Could you check a few things on this model? Use its own coordinates, in mm. Face numbers are marked on the shaded views. A direction names the side the tool comes from. Round coordinates to 2 decimals unless told otherwise and drop trailing zeros. Write each loop counter-clockwise with the first axis right and the second up, starting at its lowest first coordinate (ties: lowest second). Pieces come first, ordered by that corner, then holes. Notation, with made-up numbers: (-31, -18.5) -> (-10, -18.5) arc R13 cw to (-10, -4.5) -> close; hole circle Ø9 at (-30, 34). An arc over 180 degrees is marked (long way). Answer in a Markdown table with one row per item.
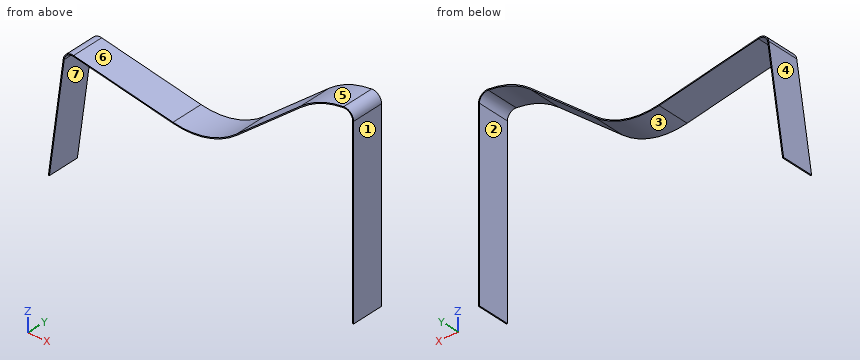
from build123d import *

# Parameters (mm, degrees)
F1_DEPTH      = 25.4
F1_DEPTH_BACK = 25.4


with BuildPart() as f1:
    # F0 (on Front) → F1 (new body, two sides)
    with BuildSketch(Plane.XZ) as f1_sk:
        with BuildLine():
            Line((-1.560986, 0.208131), (0, 0))
            Line((0, 0), (23.665896, 177.494217))
            ThreePointArc((23.665896, 177.494217), (28.705317, 186.028474), (38.342357, 188.34294))
            Line((38.342357, 188.34294), (196.490305, 161.984949))
            ThreePointArc((196.490305, 161.984949), (250.659549, 164.697858), (298.757135, 189.763554))
            Line((298.757135, 189.763554), (401.211842, 275.293424))
            ThreePointArc((401.211842, 275.293424), (432.73779, 294.602226), (468.488889, 304.013615))
            ThreePointArc((468.488889, 304.013615), (478.366667, 300.858274), (482.6, 291.392253))
            Line((482.6, 291.392253), (482.6, 0))
            Line((482.6, 0), (484.1748, 0))
            Line((484.1748, 0), (484.1748, 291.392253))
            ThreePointArc((484.1748, 291.392253), (479.416533, 302.032061), (468.313911, 305.578664))
            ThreePointArc((468.313911, 305.578664), (432.119499, 296.050574), (400.202629, 276.502342))
            Line((400.202629, 276.502342), (297.747922, 190.972472))
            ThreePointArc((297.747922, 190.972472), (250.246746, 166.217591), (196.749201, 163.538322))
            Line((196.749201, 163.538322), (38.601253, 189.896314))
            ThreePointArc((38.601253, 189.896314), (27.769219, 187.294853), (22.10491, 177.702348))
            Line((22.10491, 177.702348), (-1.560986, 0.208131))
        make_face()
    extrude(amount=F1_DEPTH)
    extrude(f1_sk.sketch, amount=-F1_DEPTH_BACK)


solid = f1.part
1) Thinking about a two-plate mould opening in X: for the marked faces 1, 2, 3 and 4, which applies, +X half, -X half, draft (parallel to the pull), parting line (faces both ways), or undercut?
Findings:
| item | result |
|---|---|
| face 1 | +X half |
| face 2 | undercut |
| face 3 | undercut |
| face 4 | -X half |
2) Imagine slicing it at C-C, the plane z = 78. Please give me the cut outline in (x, y).
Findings:
| item | result |
|---|---|
| outline | (8.81, -25.4) -> (10.4, -25.4) -> (10.4, 25.4) -> (8.81, 25.4) -> close; (482.6, -25.4) -> (484.17, -25.4) -> (484.17, 25.4) -> (482.6, 25.4) -> close |
3) Imagine slicing it at B-B, the plane y = -14. Please give me the cut outline in (x, z).
Findings:
| item | result |
|---|---|
| outline | (-1.56, 0.21) -> (0, 0) -> (23.67, 177.49) arc R12.7 cw to (38.34, 188.34) -> (196.49, 161.98) arc R127 ccw to (298.76, 189.76) -> (401.21, 275.29) arc R127 cw to (468.49, 304.01) arc R12.7 cw to (482.6, 291.39) -> (482.6, 0) -> (484.17, 0) -> (484.17, 291.39) arc R14.27 ccw to (468.31, 305.58) arc R128.57 ccw to (400.2, 276.5) -> (297.75, 190.97) arc R125.43 cw to (196.75, 163.54) -> (38.6, 189.9) arc R14.27 ccw to (22.1, 177.7) -> close |
4) Please list where these lines run through material, in increasing order: line 1 (Z direction, x = 215.5, y = 3); line 2 (Z direction, x = 197, y = 16); line 3 (X direction, y = -16, z = 236).
Findings:
| item | result |
|---|---|
| line 1 | z = 160.27 to 161.85 |
| line 2 | z = 161.9 to 163.5 |
| line 3 | x = 351.69 to 354.14, 482.6 to 484.17 |
5) Imagine slicing it at A-A, the plane z = 200.5. Please give me the cut outline in (x, y), plus the area to 3 significant figures.
Findings:
| item | result |
|---|---|
| outline | (309.16, -25.4) -> (311.62, -25.4) -> (311.62, 25.4) -> (309.16, 25.4) -> close; (482.6, -25.4) -> (484.17, -25.4) -> (484.17, 25.4) -> (482.6, 25.4) -> close |
| area | 205 mm^2 |
6) For pin 1 (2 mm diameter, centred on x = 149, y = 11.5, fed in from +Z); pin 2 (12 mm diameter, centred on x = 344, y = 16.5, fed in from -Z), each with a flat end and sliding along its axis, tell me the tip position at first contact or that it passes through.
Findings:
| item | result |
|---|---|
| pin 1 | stops at z = 171.66 |
| pin 2 | stops at z = 222.52 |
7) For the marked faces 5, 6 and 7, which set-ups out of +Z, -Z, +X, -X, +Y, -Y let a thin tool reach every point of the face, with its end or its side?
Findings:
| item | result |
|---|---|
| face 5 | +Z, -X, +Y, -Y |
| face 6 | +Z, +Y, -Y |
| face 7 | -Z, +Y, -Y |
8) Imagine slicing it at D-D, the plane x = 230. Please give me the cut outline in (y, z).
Findings:
| item | result |
|---|---|
| outline | (-25.4, 160.89) -> (25.4, 160.89) -> (25.4, 162.47) -> (-25.4, 162.47) -> close |
